from build123d import *

# Parameters (mm, degrees)
SKETCH1_W               = 172
SKETCH1_H               = 172
BOSS_EXTRUDE1_DEPTH     = 86
SKETCH3_R               = 3.5687
CUT_EXTRUDE1_DEPTH      = 87
CUT_EXTRUDE1_DEPTH_BACK = 87


with BuildPart() as part:
    # Sketch1 → Boss-Extrude1 (new body)
    with BuildSketch(Plane(origin=(0, 0, 0), x_dir=(1, 0, 0), z_dir=(0, 1, 0))):
        Rectangle(SKETCH1_W, SKETCH1_H)
    extrude(amount=-BOSS_EXTRUDE1_DEPTH)

    # Sketch2 → Cut-Revolve1 (revolve, cut)
    with BuildSketch(Plane.XY):
        with BuildLine():
            Line((0, -35), (0, 0))
            Line((0, 0), (35, 0))
            ThreePointArc((35, 0), (24.748737342, -24.748737342), (0, -35))
        make_face()
    revolve(axis=Axis((0, -35, 0), (0, 1, 0)), mode=Mode.SUBTRACT)

    # Sketch3 → Cut-Extrude1 (cut, two sides)
    with BuildSketch(Plane(origin=(0, 0, 0), x_dir=(0, 0, -1), z_dir=(1, 0, 0))) as cut_extrude1_sk:
        with Locations((0, -69.85)):
            Circle(SKETCH3_R)
        with Locations((69.85, -69.85)):
            Circle(SKETCH3_R)
    extrude(amount=CUT_EXTRUDE1_DEPTH, mode=Mode.SUBTRACT)
    extrude(cut_extrude1_sk.sketch, amount=-CUT_EXTRUDE1_DEPTH_BACK, mode=Mode.SUBTRACT)


solid = part.part
Geometry: final body of the model. Coordinates: model frame, mm. Give positions to 0.01 mm unless a question says otherwise; leave off trailing zeros. Loops run counter-clockwise (first coordinate to the right, second up) from the corner with the lowest first, then second, coordinate; pieces in that order, holes last. Notation, with made-up numbers: (21, 83.25) - (71, 83.25) arc R20 ccw to (71, 122.25) - close; hole circle Ø2 at (-39, 8.25). An arc over 180 degrees is marked (long way). Answer as CSV lines item,"result". Start each with the question number.
1. Section D-D, the plane z = 14. Return loops of the section in (x, y).
2. Section C-C, the plane y = -19.5. Return loops of the section in (x, z), plus the area to 3 significant figures.
3. Pin query (flat end, axial travel): P1, Ø1.5, axis at x = -53, z = -42, coming from the +Y side. Return the tip coordinate at first contact, or that it passes through.
4. Section B-B, the plane z = -69.85. Return loops of the section in (x, y).
5. Draft query along Z for faces 1 (the face through (-1, -42, 86)), 2 (the face through (37, 0, -1)), 3 (the face through (1.204, -73.016, -1.647)), 4 (the face through (-1, -42, -86)). Return one class per face: released by +Z, released by -Z, zero draft, split by the parting line, or undercut.
6. Section A-A, the plane y = -69.85. Return loops of the section in (x, z), plus the area to 3 significant figures.
7. Ray query, L1, parallel to Z at x = 33, y = -69.85; L2, parallel to Y at x = -16, z = -69.85; L3, parallel to Z at x = 1, y = -69. Return the intervals inside material, ascending.
Answers:
1,outline,"(-86, -86) - (86, -86) - (86, 0) - (32.08, 0) arc R32.08 cw to (-32.08, 0) - (-86, 0) - close"
2,outline,"(-86, -86) - (86, -86) - (86, 86) - (-86, 86) - close; hole circle Ø58.13 at (0, 0)"
2,area,"26,900 mm2"
3,P1,"stops at y = 0"
4,outline,"(-86, -86) - (86, -86) - (86, -73.42) - (-86, -73.42) - close; (-86, -66.28) - (86, -66.28) - (86, 0) - (-86, 0) - close"
5,face 1,"released by +Z"
5,face 2,"zero draft"
5,face 3,"undercut"
5,face 4,"released by -Z"
6,outline,"(-86, -86) - (86, -86) - (86, -73.42) - (-86, -73.42) - close; (-86, -66.28) - (86, -66.28) - (86, -3.57) - (-86, -3.57) - close; (-86, 3.57) - (86, 3.57) - (86, 86) - (-86, 86) - close"
6,area,"27,100 mm2"
7,L1,"z = -86 to -73.42, -66.28 to -3.57, 3.57 to 86"
7,L2,"y = -86 to -73.42, -66.28 to 0"
7,L3,"z = -86 to -73.32, -66.38 to -3.47, 3.47 to 86"
